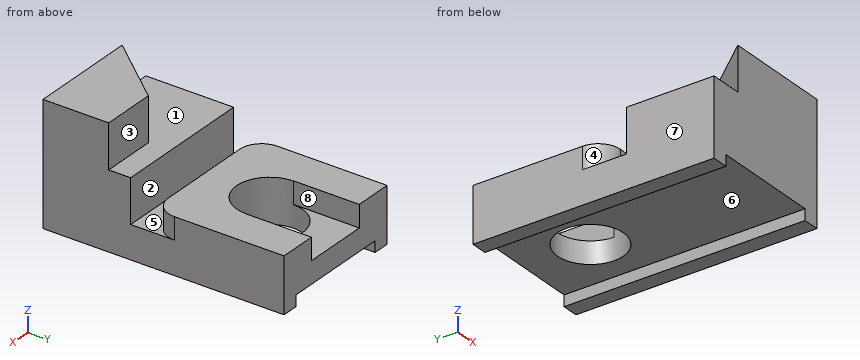
from build123d import *

# Parameters (mm, degrees)
ESBO_O1_W                = 130
ESBO_O1_H                = 80
RESSALTO_EXTRUS_O1_DEPTH = 70
RESSALTO_EXTRUS_O2_DEPTH = 40
ESBO_O3_W                = 130
ESBO_O3_H                = 30.168266629
RESSALTO_EXTRUS_O3_DEPTH = 140
ESBO_O4_W                = 130
ESBO_O4_H                = 120
RESSALTO_EXTRUS_O4_DEPTH = 20
ESBO_O5_W                = 100
ESBO_O5_H                = 10
CORTE_EXTRUS_O1_DEPTH    = 260
FILETE3_R                = 20
FILETE4_R                = 20
ESBO_O12_W               = 60.538405015
ESBO_O12_H               = 20.084133314
CORTE_EXTRUS_O3_DEPTH    = 60
ESBO_O13_R               = 30
CORTE_EXTRUS_O4_DEPTH    = 60


with BuildPart() as part:
    # Esboço1 → Ressalto-extrusão1 (new body)
    with BuildSketch(Plane.XY):
        with Locations((65, 40)):
            Rectangle(ESBO_O1_W, ESBO_O1_H)
    extrude(amount=RESSALTO_EXTRUS_O1_DEPTH)

    # Esboço2 → Ressalto-extrusão2 (add)
    with BuildSketch(Plane.XY.offset(70)):
        Polygon((130, 0), (30, 0), (80, 60.000756035), (130, 60.000756035), align=None)
    extrude(amount=RESSALTO_EXTRUS_O2_DEPTH)

    # Esboço3 → Ressalto-extrusão3 (add)
    with BuildSketch(Plane(origin=(0, 80, 0), x_dir=(1, 0, 0), z_dir=(0, 1, 0))):
        with Locations((65, -15.084133315)):
            Rectangle(ESBO_O3_W, ESBO_O3_H)
    extrude(amount=RESSALTO_EXTRUS_O3_DEPTH)

    # Esboço4 → Ressalto-extrusão4 (add)
    with BuildSketch(Plane.XY.offset(30.168266629)):
        with Locations((65, 160)):
            Rectangle(ESBO_O4_W, ESBO_O4_H)
    extrude(amount=RESSALTO_EXTRUS_O4_DEPTH)

    # Esboço5 → Corte-extrusão1 (cut)
    with BuildSketch(Plane(origin=(0, 220, 0), x_dir=(1, 0, 0), z_dir=(0, 1, 0))):
        with Locations((65, -5)):
            Rectangle(ESBO_O5_W, ESBO_O5_H)
    extrude(amount=-CORTE_EXTRUS_O1_DEPTH, mode=Mode.SUBTRACT)

    # Filete3
    filete3_edges = [part.edges().sort_by_distance(p)[0] for p in [
        (0, 100, 40.168266629),
    ]]
    fillet(filete3_edges, radius=FILETE3_R)

    # Filete4
    filete4_edges = [part.edges().sort_by_distance(p)[0] for p in [
        (130, 100, 40.168266629),
    ]]
    fillet(filete4_edges, radius=FILETE4_R)

    # Esboço12 → Corte-extrusão3 (cut)
    with BuildSketch(Plane(origin=(0, 220, 0), x_dir=(1, 0, 0), z_dir=(0, 1, 0))):
        with Locations((65.269202508, -40.126199972)):
            Rectangle(ESBO_O12_W, ESBO_O12_H)
    extrude(amount=-CORTE_EXTRUS_O3_DEPTH, mode=Mode.SUBTRACT)

    # Esboço13 → Corte-extrusão4 (cut)
    with BuildSketch(Plane.XY.offset(50.168266629)):
        with Locations((65.269202508, 160)):
            Circle(ESBO_O13_R)
    extrude(amount=-CORTE_EXTRUS_O4_DEPTH, mode=Mode.SUBTRACT)


solid = part.part
Input: part model. Units: mm. Frame: model coordinates. Face numbers are marked on the shaded views. A direction names the side the tool comes from. Give positions to 0.01 mm unless a question says otherwise; leave off trailing zeros. Write each loop counter-clockwise with the first axis right and the second up, starting at its lowest first coordinate (ties: lowest second). Pieces come first, ordered by that corner, then holes.
Q1. Section C-C, the plane z = 17.5. Output: boundary loops of the cut face in (x, y), plus the area to 3 significant figures.
Q2. Pull-direction query (X, two-part tool) for the marked faces 5, 6, 7 and 8; classes: pulls with the +X half, pulls with the -X half, needs draft (parallel to the pull), parting line crosses it, or undercut.
Q3. Section D-D, the plane y = 67.5. Output: boundary loops of the cut face in (x, z).
Q4. Section A-A, the plane x = 42.5. Output: boundary loops of the cut face in (y, z), plus the area to 3 significant figures.
Q5. Set-up query: the marked faces 1, 2, 3 and 4. Return all of +Z, -Z, +X, -X, +Y, -Y with unobstructed straight access to the full face (end or side cutting, diameter ignored); none if empty.
Q6. First-contact query: P1, Ø5, axis at x = 35.5, y = 103, coming from the +Z side; P2, Ø10, axis at x = 80, z = 37.5, coming from the -Y side; P3, Ø1.5, axis at x = 58, y = 23, coming from the -Z side; P4, Ø12, axis at x = 81, z = 53.5, coming from the +Y side. Flat tips, straight axial feed; report the tip coordinate or a pass-through.
Q7. Material intervals for probe 1 along X at (y, z) = (160, 20.5); probe 2 along X at (y, z) = (161.5, 12); probe 3 along Z at (x, y) = (13, 207.5), sorted ascending.
Q8. Section B-B, the plane y = 149. Output: boundary loops of the cut face in (x, z), plus the area to 3 significant figures.
Filled in:
1. outline: (0, 0) - (130, 0) - (130, 220) - (0, 220) - close; hole circle Ø60 at (65.27, 160)
1. area: 25,800 mm2
2. face 5: needs draft
2. face 6: undercut
2. face 7: pulls with the -X half
2. face 8: undercut
3. outline: (0, 0) - (15, 0) - (15, 10) - (115, 10) - (115, 0) - (130, 0) - (130, 70) - (0, 70) - close
4. outline: (0, 10) - (140.47, 10) - (140.47, 50.17) - (100, 50.17) - (100, 30.17) - (80, 30.17) - (80, 70) - (15, 70) - (15, 110) - (0, 110) - close; (179.53, 10) - (220, 10) - (220, 30.08) - (179.53, 30.08) - close
4. area: 8,240 mm2
5. face 1: +Z, -X, +Y
5. face 2: +Z, +X, -X
5. face 3: +Z, +X, -X, +Y
5. face 4: +Z, -X
6. P1: stops at z = 50.17
6. P2: stops at y = 0
6. P3: stops at z = 10
6. P4: stops at y = 138.31
7. probe 1: x = 0 to 35.27, 95.27 to 130
7. probe 2: x = 0 to 35.31, 95.23 to 130
7. probe 3: z = 0 to 50.17
8. outline: (0, 0) - (15, 0) - (15, 10) - (37.36, 10) - (37.36, 50.17) - (0, 50.17) - close; (93.18, 10) - (115, 10) - (115, 0) - (130, 0) - (130, 50.17) - (93.18, 50.17) - close
8. area: 3,280 mm2
